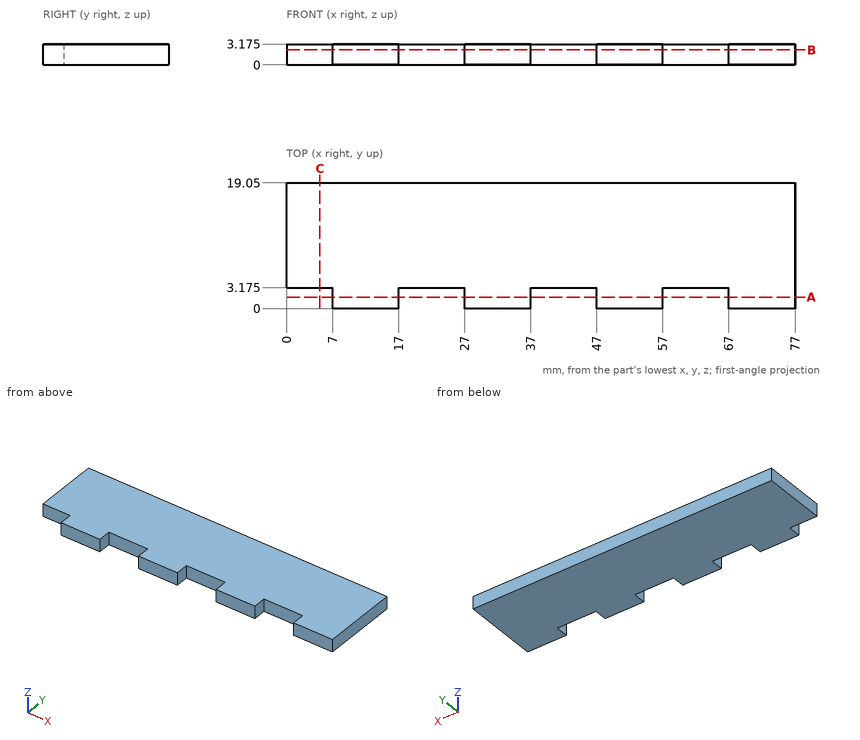
Input: dimensioned drawing with shaded views. Units: mm. Origin: part minimum x, y, z. Coordinates: 2 decimals unless noted, no trailing zeros. Write each loop counter-clockwise with the first axis right and the second up, starting at its lowest first coordinate (ties: lowest second). Pieces come first, ordered by that corner, then holes. Notation, with made-up numbers: M -5.5,-8.75 L 49.5,-8.75 A12 ccw 49.5,7.25 Z; hole C 76.25,-11.5 d5. An arc over 180 degrees is marked long. Use a Markdown table: item, result.
1) Section A-A, the plane y = 1.75. Output: boundary loops of the cut face in (x, z) (3 decimals), then the cut area to 3 significant figures.
Conclusion:
| item | result |
|---|---|
| outline | M 7,0 L 17,0 L 17,3.175 L 7,3.175 Z; M 27,0 L 37,0 L 37,3.175 L 27,3.175 Z; M 47,0 L 57,0 L 57,3.175 L 47,3.175 Z; M 67,0 L 77,0 L 77,3.175 L 67,3.175 Z |
| area | 127 mm^2 |
2) Section C-C, the plane x = 5. Output: boundary loops of the cut face in (y, z) (3 decimals), then the cut area to 3 significant figures.
Conclusion:
| item | result |
|---|---|
| outline | M 3.175,0 L 19.05,0 L 19.05,3.175 L 3.175,3.175 Z |
| area | 50.4 mm^2 |
3) Section B-B, the plane z = 2.3. Output: boundary loops of the cut face in (x, y) (3 decimals), then the cut area to 3 significant figures.
Conclusion:
| item | result |
|---|---|
| outline | M 0,3.175 L 7,3.175 L 7,0 L 17,0 L 17,3.175 L 27,3.175 L 27,0 L 37,0 L 37,3.175 L 47,3.175 L 47,0 L 57,0 L 57,3.175 L 67,3.175 L 67,0 L 77,0 L 77,19.05 L 0,19.05 Z |
| area | 1,350 mm^2 |
4) Ray query, L1, parallel to X at y = 1.75, z = 1.8; L2, parallel to Y at x = 24, z = 2.85 (3 decimals). Return the intervals inside material, ascending.
Conclusion:
| item | result |
|---|---|
| L1 | x = 7 to 17, 27 to 37, 47 to 57, 67 to 77 |
| L2 | y = 3.175 to 19.05 |
5) First-contact query: pin 1 Ø1 at (x, z) = (41, 1.5) entering from -Y (3 decimals); pin 2 Ø1 at (y, z) = (1, 2.5) entering from -X. Flat tips, straight axial feed; report the tip coordinate or a pass-through.
Conclusion:
| item | result |
|---|---|
| pin 1 | stops at y = 3.175 |
| pin 2 | stops at x = 7 |
